Here's how the part is built. I have some questions about the finished solid (model axes, mm). A direction names the side the tool comes from. Round coordinates to 2 decimals unless told otherwise and drop trailing zeros. Loops run counter-clockwise (first coordinate to the right, second up) from the corner with the lowest first, then second, coordinate; pieces in that order, holes last. Notation, with made-up numbers: M -16.75,21.5 L 31.25,21.5 A29 cw 31.25,41.5 Z; hole C 32,21 d10. An arc over 180 degrees is marked long. Answer as a JSON object with one key per item and string values.
from build123d import *

# Parameters (mm, degrees)
F0_R      = 22.5
F1_DEPTH  = 300
F2_W      = 24.0328347509
F2_H      = 38.0450108928
F3_DEPTH  = 25.4
F4_W      = 38.0450108928
F4_H      = 25.4
F5_DEPTH  = 250
F6_W      = 50
F6_H      = 38.0450108928
F7_DEPTH  = 75
F9_W      = 38.0450108928
F9_H      = 25.4
F10_DEPTH = 250
F11_W     = 50
F11_H     = 38.0450108928
F12_DEPTH = 75
F13_R     = 16.7747006108
F14_DEPTH = 150
F8_R      = 17.5763954382
F15_DEPTH = 150
F16_SIZE  = 5.08


with BuildPart() as f1:
    # F0 (on Top) → F1 (new body)
    with BuildSketch(Plane.XY):
        with Locations((-6.6593382508, 15.5711015686)):
            Circle(F0_R)
    extrude(amount=F1_DEPTH)

    # F2 (on face) → F3 (join)
    with BuildSketch(Plane.XY.offset(300)):
        with Locations((-6.6593382508, 15.5711015686)):
            Rectangle(F2_W, F2_H)
    extrude(amount=F3_DEPTH)

    # F4 (on face) → F5 (join)
    with BuildSketch(Plane(origin=(-18.6757556262, 0, 0), x_dir=(0, -1, 0), z_dir=(-1, 0, 0))):
        with Locations((-15.5711015686, 312.7)):
            Rectangle(F4_W, F4_H)
    extrude(amount=F5_DEPTH)

    # F6 (on face) → F7 (join)
    with BuildSketch(Plane.XY.offset(325.4)):
        with Locations((-243.6757556262, 15.5711015686)):
            Rectangle(F6_W, F6_H)
    extrude(amount=F7_DEPTH)

    # F9 (on face) → F10 (join)
    with BuildSketch(Plane.YZ.offset(5.3570791247)):
        with Locations((15.5711015686, 312.7)):
            Rectangle(F9_W, F9_H)
    extrude(amount=F10_DEPTH)

    # F11 (on face) → F12 (join)
    with BuildSketch(Plane.XY.offset(325.4)):
        with Locations((230.3570791247, 15.5711015686)):
            Rectangle(F11_W, F11_H)
    extrude(amount=F12_DEPTH)

    # F13 (on face) → F14 (join)
    with BuildSketch(Plane.YZ.offset(255.3570791247)):
        with Locations((15.5711015686, 380.4)):
            Circle(F13_R)
    extrude(amount=F14_DEPTH)

    # F8 (on face) → F15 (join)
    with BuildSketch(Plane(origin=(-268.6757556262, 0, 0), x_dir=(0, -1, 0), z_dir=(-1, 0, 0))):
        with Locations((-16.2542480975, 380.010843277)):
            Circle(F8_R)
    extrude(amount=F15_DEPTH)

    # F16
    f16_edges = [f1.edges().sort_by_distance(p)[0] for p in [
        (-6.659338, -3.451404, 325.4),
        (-6.659338, 34.593607, 325.4),
        (-218.675756, -3.451404, 362.9),
        (-218.675756, 34.593607, 362.9),
        (205.357079, -3.451404, 362.9),
        (205.357079, 34.593607, 362.9),
        (205.357079, 15.571102, 400.4),
        (-218.675756, 15.571102, 400.4),
        (-243.675756, -3.451404, 400.4),
        (-243.675756, 34.593607, 400.4),
        (230.357079, 34.593607, 400.4),
        (230.357079, -3.451404, 400.4),
    ]]
    chamfer(f16_edges, length=F16_SIZE)


solid = f1.part
Item 1: I want a section at C-C on x = 307. List the corners of the cut face in (y, z) for me.
Solution:
{"outline": "C 15.57,380.4 d33.55"}
Item 2: We'd pull the mould along X, two halves only. Please class faces 1 (the face through (-7, 16, 0)), 2 (the face through (-10, 15, 325.4)), 3 (the face through (205.357, 15, 360)), 4 (the face through (405.357, 15, 381)): +X half, -X half, draft (parallel to the pull), parting line (faces both ways), or undercut.
Solution:
{"face 1": "draft", "face 2": "undercut", "face 3": "undercut", "face 4": "+X half"}
Item 3: For faces 5 (the face through (-218.676, 15, 360)), 6 (the face through (-342.63, 20.06, 362.85)), 7 (the face through (329.307, 11.935, 364.024)), 8 (the face through (-11.5, -6.4, 147.9)), which set-ups out of +Z, -Z, +X, -X, +Y, -Y let a thin tool reach every point of the face, with its end or its side?
Solution:
{"face 5": "+Z, +Y, -Y", "face 6": "-X", "face 7": "+X", "face 8": "-Z"}
Item 4: I want a section at A-A on x = -143. List the corners of the cut face in (y, z) for me, plus the area to 3 significant figures.
Solution:
{"outline": "M -3.45,300 L 34.59,300 L 34.59,320.32 L 29.51,325.4 L 1.63,325.4 L -3.45,320.32 Z", "area": "941 mm2"}
Item 5: If I drill on L1, parallel to X at y = 14.5, z = 376; L2, parallel to X at y = 16.5, z = 149; L3, parallel to X at y = 26, z = 356, over which ranges is the centre line in solid material (lowest first)? Write a range as from..to.
Solution:
{"L1": "x = -418.68..-218.68, 205.36..405.36", "L2": "x = -29.14..15.82", "L3": "x = -268.68..-218.68, 205.36..255.36"}
Item 6: For P1, Ø19, axis at x = -89, y = 10, coming from the -Z side; P2, Ø1, axis at y = 31, z = 274.5, coming from the -X side; P3, Ø10, axis at y = 1.5, z = 161, coming from the +X side, each with a flat end and sliding along its axis, tell me the tip position at first contact or that it passes through.
Solution:
{"P1": "stops at z = 300", "P2": "stops at x = -23.49", "P3": "stops at x = 13.93"}
Item 7: I want a section at B-B on z = 110.5. List the corners of the cut face in (x, y) for me, plus the area to 3 significant figures.
Solution:
{"outline": "C -6.66,15.57 d45", "area": "1,590 mm2"}
